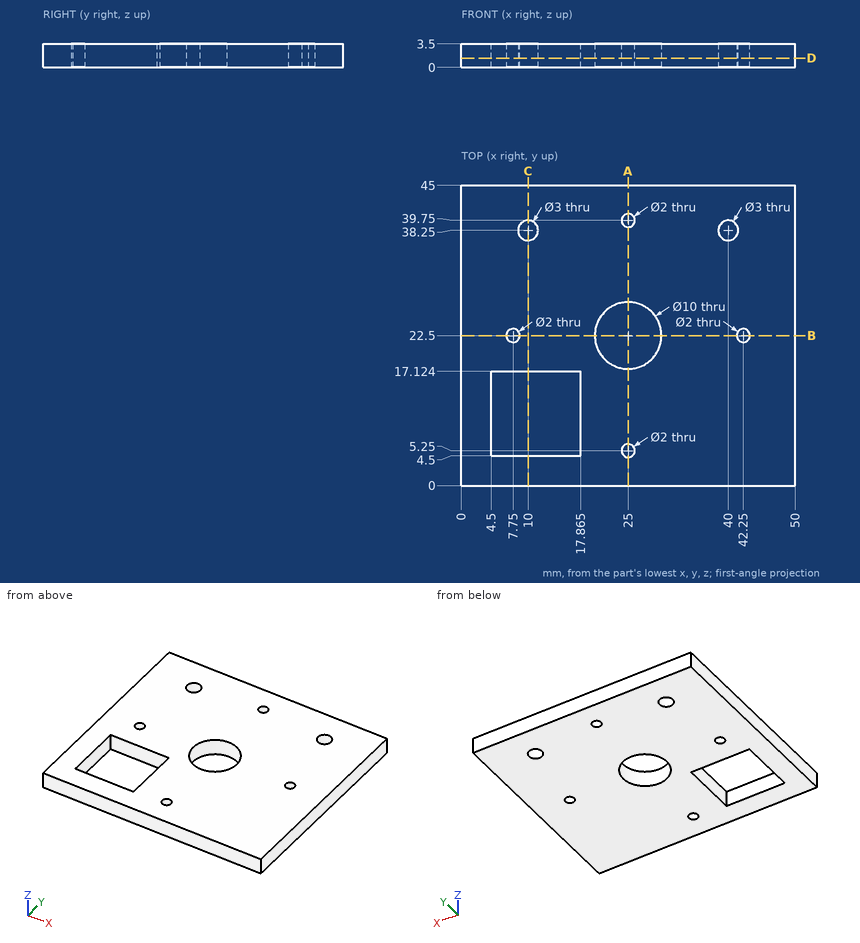
Answer from the drawing. Dimensions are ordinates in mm from the lowest x, y and z of the part. Coordinates: 2 decimals unless noted, no trailing zeros. Write each loop counter-clockwise with the first axis right and the second up, starting at its lowest first coordinate (ties: lowest second). Pieces come first, ordered by that corner, then holes. Notation, with made-up numbers: M 88.25,58.5 L 109.25,58.5 A34 cw 109.25,90.5 Z; hole C 25,15 d11. An arc over 180 degrees is marked long. Put each result on its own line as item: value. Start each with the question number.
1. A flat-ended cylindrical pin translates along its axis: P1, Ø1.5, axis at x = 29.5, y = 15, coming from the -Z side. Find the tip coordinate at first contact, or state that the pin passes through.
2. Consider line 1 (Y direction, x = 25, z = 2.85); line 2 (Y direction, x = 7.75, z = 2.6); line 3 (X direction, y = 7, z = 2.2) (1 decimal). Determine where each line is inside the solid, lowest interval first. Write a range as from..to.
3. A cutting plane is placed at B-B on y = 22.5. Write down the section's boundary in (x, z), then the cut area to 3 significant figures.
4. A cutting plane is placed at D-D on z = 1.4. Count the separate pieces of the cut face and the enclosed holes in it, then the cut area to 3 significant figures.
5. A cutting plane is placed at C-C on x = 10. Write down the section's boundary in (y, z).
6. A cutting plane is placed at A-A on x = 25. Write down the section's boundary in (y, z).
Resolved:
1. P1: stops at z = 0
2. line 1: y = 0..4.25, 6.25..17.5, 27.5..38.75, 40.75..45
2. line 2: y = 0..4.5, 17.12..21.5, 23.5..45
2. line 3: x = 0..4.5, 17.9..50
3. outline: M 0,0 L 6.75,0 L 6.75,3.5 L 0,3.5 Z; M 8.75,0 L 20,0 L 20,3.5 L 8.75,3.5 Z; M 30,0 L 41.25,0 L 41.25,3.5 L 30,3.5 Z; M 43.25,0 L 50,0 L 50,3.5 L 43.25,3.5 Z
3. area: 126 mm2
4. separate pieces: 1
4. enclosed holes: 8
4. area: 1,980 mm2
5. outline: M 0,0 L 4.5,0 L 4.5,3.5 L 0,3.5 Z; M 17.12,0 L 36.75,0 L 36.75,3.5 L 17.12,3.5 Z; M 39.75,0 L 45,0 L 45,3.5 L 39.75,3.5 Z
6. outline: M 0,0 L 4.25,0 L 4.25,3.5 L 0,3.5 Z; M 6.25,0 L 17.5,0 L 17.5,3.5 L 6.25,3.5 Z; M 27.5,0 L 38.75,0 L 38.75,3.5 L 27.5,3.5 Z; M 40.75,0 L 45,0 L 45,3.5 L 40.75,3.5 Z
